Geometry: final body of the model. Coordinates: model frame, mm. A direction names the side the tool comes from. Give positions to 0.01 mm unless a question says otherwise; leave off trailing zeros. Write each loop counter-clockwise with the first axis right and the second up, starting at its lowest first coordinate (ties: lowest second). Pieces come first, ordered by that corner, then holes. Notation, with made-up numbers: M 32,-2.5 L 84,-2.5 A17 ccw 84,7.5 Z; hole C 51.25,71.25 d4. An arc over 180 degrees is marked long. One line per question, with ' | ' between items.
from build123d import *

# Parameters (mm, degrees)
F2_R      = 4
F3_DEPTH  = 20.001
F5_R      = 23
F5_R_2    = 11
F6_DEPTH  = 3
F8_R      = 23
F8_R_2    = 11
F9_DEPTH  = 3
F10_R     = 4
F11_DEPTH = 25


with BuildPart() as f1:
    # F0 (on Front) → F1 (revolve)
    with BuildSketch(Plane.XZ):
        Polygon((10.9751848876, 5), (10.9751848876, 25), (5.9751848876, 25), (5.9751848876, 24), (-4.0248151124, 24), (-4.0248151124, 25), (-9.0248151124, 25), (-9.0248151124, 5), align=None)
    revolve(axis=Axis((1.0365527123, 0, 0), (1, 0, 0)))

    # F2 (on face) → F3 (cut, through all)
    with BuildSketch(Plane(origin=(-9.0248151124, 0, 0), x_dir=(0, -1, 0), z_dir=(-1, 0, 0))):
        with Locations((0, 15)):
            Circle(F2_R)
        with Locations((-15, 0)):
            Circle(F2_R)
        with Locations((0, -15)):
            Circle(F2_R)
    extrude(amount=-F3_DEPTH, mode=Mode.SUBTRACT)

    # F5 (on offset) → F6 (cut)
    with BuildSketch(Plane(origin=(-10.0248151124, 0, 0), x_dir=(0, -1, 0), z_dir=(-1, 0, 0))):
        Circle(F5_R)
        Circle(F5_R_2, mode=Mode.SUBTRACT)
    extrude(amount=-F6_DEPTH, mode=Mode.SUBTRACT)

    # F8 (on offset) → F9 (cut)
    with BuildSketch(Plane.YZ.offset(11.9751848876)):
        Circle(F8_R)
        Circle(F8_R_2, mode=Mode.SUBTRACT)
    extrude(amount=-F9_DEPTH, mode=Mode.SUBTRACT)

    # F10 (on face) → F11 (join)
    with BuildSketch(Plane(origin=(-7.0248151124, 0, 0), x_dir=(0, -1, 0), z_dir=(-1, 0, 0))):
        with Locations((15.1, 0)):
            Circle(F10_R)
    extrude(amount=F11_DEPTH)


solid = f1.part
(1) First-contact query: P1, Ø6.5, axis at y = 1.5, z = 3.5, coming from the -X side; P2, Ø1, axis at x = -25, y = -15.5, coming from the -Z side; P3, Ø10, axis at x = -23.5, y = -11, coming from the +Z side. Flat tips, straight axial feed; report the tip coordinate or a pass-through.
Working result:
P1: stops at x = -9.02 | P2: stops at z = -4 | P3: stops at z = 4
(2) Set-up query: faces 1 (the face through (9.989, -2.994, 22.804)), 2 (the face through (-8.039, 2.994, 22.804)), 3 (the face through (-4.025, -22.3, 9.4)). Return all of +Z, -Z, +X, -X, +Y, -Y with unobstructed straight access to the full face (end or side cutting, diameter ignored); none if empty.
Working result:
face 1: +X | face 2: -X | face 3: none
(3) Cut plane D-D, the plane x = -17. Return loops of the section in (y, z).
Working result:
outline: C -15.1,0 d8
(4) Draft query along Y for faces 4 (the face through (-32.025, -15, 0)), 5 (the face through (8.975, -5, -10)), 6 (the face through (8.44, -7.509, 23.846)). Return one class per face: released by +Y, released by -Y, zero draft, split by the parting line, or undercut.
Working result:
face 4: zero draft | face 5: undercut | face 6: split by the parting line
(5) Material intervals for L1, parallel to Z at x = 2, y = 0; L2, parallel to Z at x = -7.7, y = 0; L3, parallel to X at y = -9.5, z = 22.5, sorted ascending. Write a range as [from, to].
Working result:
L1: z = [-24, -19], [-11, -5], [5, 11], [19, 24] | L2: z = [-25, -23], [-11, -5], [5, 11], [23, 25] | L3: x = [-9.02, -4.02], [5.98, 10.98]
(6) Cut plane A-A, the plane z = -15. Return loops of the section in (x, y) (3 decimals).
Working result:
outline: M -9.025,-20 L -4.025,-20 L -4.025,-18.735 L 5.975,-18.735 L 5.975,-20 L 10.975,-20 L 10.975,-17.436 L 8.975,-17.436 L 8.975,-4 L -7.025,-4 L -7.025,-17.436 L -9.025,-17.436 Z; M -9.025,17.436 L -7.025,17.436 L -7.025,4 L 8.975,4 L 8.975,17.436 L 10.975,17.436 L 10.975,20 L 5.975,20 L 5.975,18.735 L -4.025,18.735 L -4.025,20 L -9.025,20 Z
(7) Cut plane B-B, the plane y = -15. Return loops of the section in (x, z) (3 decimals), then the cut area to 3 significant figures.
Working result:
outline: M -32.025,-3.999 L -7.025,-3.999 L -7.025,-17.436 L -9.025,-17.436 L -9.025,-20 L -4.025,-20 L -4.025,-18.735 L 5.975,-18.735 L 5.975,-20 L 10.975,-20 L 10.975,-17.436 L 8.975,-17.436 L 8.975,17.436 L 10.975,17.436 L 10.975,20 L 5.975,20 L 5.975,18.735 L -4.025,18.735 L -4.025,20 L -9.025,20 L -9.025,17.436 L -7.025,17.436 L -7.025,3.999 L -32.025,3.999 Z | area: 835 mm^2
(8) Cut plane C-C, the plane z = 10. Return loops of the section in (x, y).
Working result:
outline: M -9.02,-22.91 L -4.02,-22.91 L -4.02,-21.82 L 5.98,-21.82 L 5.98,-22.91 L 10.98,-22.91 L 10.98,-20.71 L 8.98,-20.71 L 8.98,-4.58 L 10.98,-4.58 L 10.98,4.58 L 8.98,4.58 L 8.98,20.71 L 10.98,20.71 L 10.98,22.91 L 5.98,22.91 L 5.98,21.82 L -4.02,21.82 L -4.02,22.91 L -9.02,22.91 L -9.02,20.71 L -7.02,20.71 L -7.02,4.58 L -9.02,4.58 L -9.02,-4.58 L -7.02,-4.58 L -7.02,-20.71 L -9.02,-20.71 Z
